Verification items for this drawing (mm, ordinates from the low corner). Round coordinates to 2 decimals unless told otherwise and drop trailing zeros. Loops run counter-clockwise (first coordinate to the right, second up) from the corner with the lowest first, then second, coordinate; pieces in that order, holes last. Notation, with made-up numbers: M 45.5,18.25 L 93.5,18.25 A23 cw 93.5,37.25 Z; hole C 24,-32 d5. An arc over 180 degrees is marked long. Answer in a Markdown table with one row per item. Add a question column.
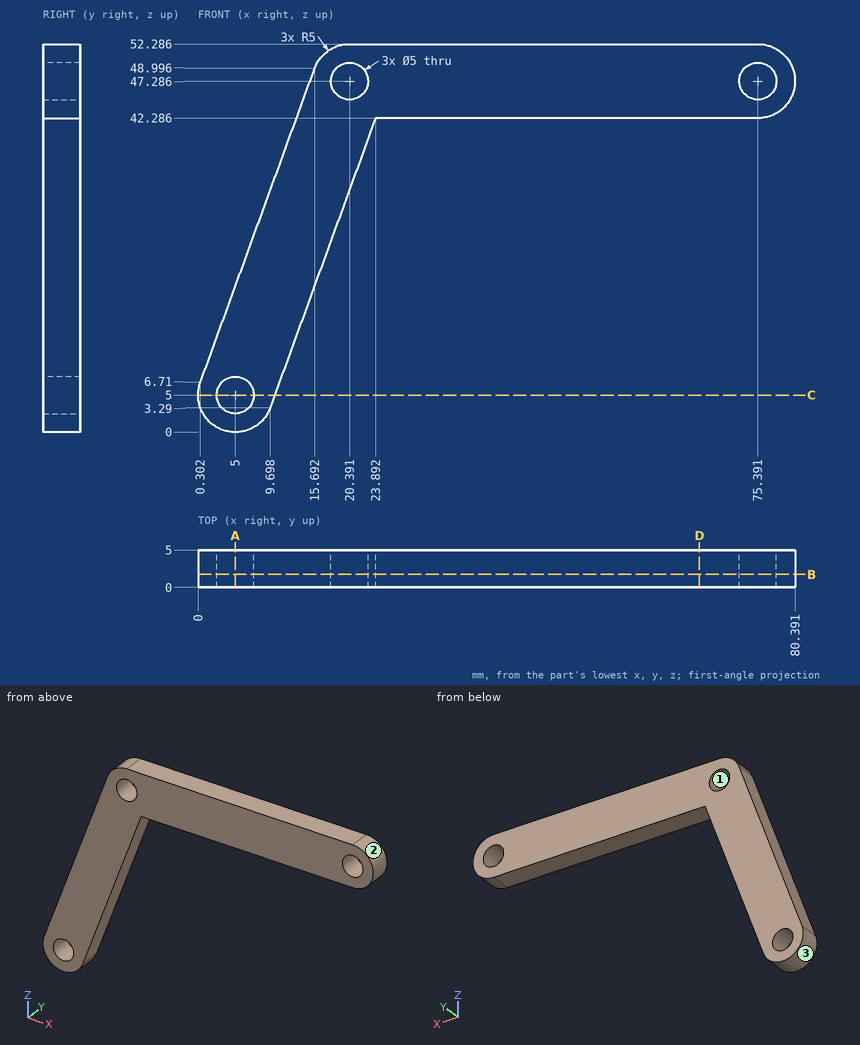
1) Cross-section at D-D, the plane x = 67.5. Record the boundary of the cut face in (y, z).
2) Cross-section at B-B, the plane y = 1.75. Record the boundary of the cut face in (x, z), plus the area to 3 significant figures.
3) Draft check along X on the marked faces 1, 2 and 3. Enter one of: +X half, -X half, draft (parallel to the pull), parting line (faces both ways), or undercut.
4) Go/stop test with flat-tipped pins: pin 1 (2 mm diameter, centred on y = 1.5, z = 36, fed in from -X); pin 2 (2 mm diameter, centred on y = 4, z = 11.5, fed in from +X). Record where each tip stops, or that it passes through.
5) Cross-section at C-C, the plane z = 5. Record the boundary of the cut face in (x, y), plus the area to 3 significant figures.
6) Cross-section at A-A, the plane x = 5. Record the boundary of the cut face in (y, z).
7) Thickness scan on L1, parallel to X at y = 3, z = 49 (1 decimal); L2, parallel to Z at x = 71, y = 1.05; L3, parallel to X at y = 3.35, z = 6.5 (1 decimal). Record the ranges inside material, lowest first. Write a range as [from, to].
Worked answers:
| question | item | result |
|---|---|---|
| 1 | outline | M 0,42.29 L 5,42.29 L 5,52.29 L 0,52.29 Z |
| 2 | outline | M 0.3,6.71 A5 ccw 9.7,3.29 L 23.89,42.29 L 75.39,42.29 A5 ccw 75.39,52.29 L 20.39,52.29 A5 ccw 15.69,49 Z; hole C 5,5 d5; hole C 20.39,47.29 d5; hole C 75.39,47.29 d5 |
| 2 | area | 1,020 mm2 |
| 3 | face 1 | undercut |
| 3 | face 2 | +X half |
| 3 | face 3 | parting line |
| 4 | pin 1 | stops at x = 10.6 |
| 4 | pin 2 | stops at x = 13.05 |
| 5 | outline | M 0,0 L 2.5,0 L 2.5,5 L 0,5 Z; M 7.5,0 L 10.32,0 L 10.32,5 L 7.5,5 Z |
| 5 | area | 26.6 mm2 |
| 6 | outline | M 0,0 L 5,0 L 5,2.5 L 0,2.5 Z; M 0,7.5 L 5,7.5 L 5,19.62 L 0,19.62 Z |
| 7 | L1 | x = [15.7, 18.6], [22.2, 73.6], [77.2, 80.1] |
| 7 | L2 | z = [42.29, 52.29] |
| 7 | L3 | x = [0.2, 3], [7, 10.9] |
